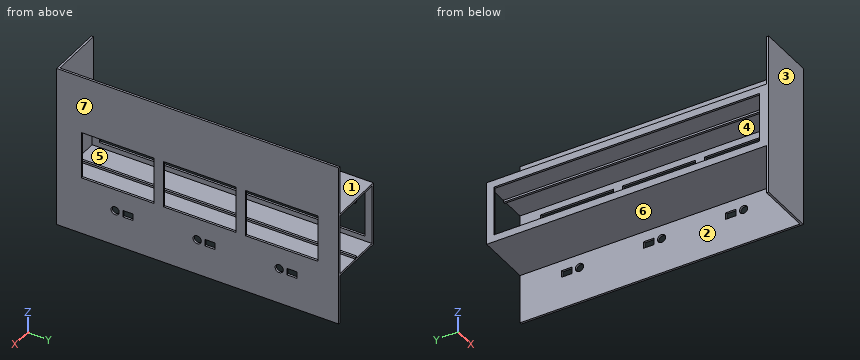
from build123d import *

# Parameters (mm, degrees)
ESQUISSE1_W             = 102
ESQUISSE1_H             = 546
BOSS_EXTRU_1_DEPTH      = 125
ESQUISSE2_W             = 117
ESQUISSE2_H             = 546
ENL_V_MAT_EXTRU_1_DEPTH = 570.3373341
ESQUISSE3_W             = 4
ESQUISSE3_H             = 546
BOSS_EXTRU_2_DEPTH      = 4
ESQUISSE4_W             = 4
ESQUISSE4_H             = 546
BOSS_EXTRU_3_DEPTH      = 4
ESQUISSE5_W             = 125
ESQUISSE5_H             = 546
BOSS_EXTRU_4_DEPTH      = 4
ESQUISSE6_W             = 97
ESQUISSE6_H             = 518
ENL_V_MAT_EXTRU_2_DEPTH = 571.067539858
ESQUISSE7_W             = 317
ESQUISSE7_H             = 546
BOSS_EXTRU_5_DEPTH      = 4
ESQUISSE8_W             = 92
ESQUISSE8_H             = 142
ENL_V_MAT_EXTRU_3_DEPTH = 600.21365138
ESQUISSE10_W            = 13.2
ESQUISSE10_H            = 20
ENL_V_MAT_EXTRU_4_DEPTH = 600.21365138
ESQUISSE12_R            = 8
ENL_V_MAT_EXTRU_5_DEPTH = 600.21365138
ESQUISSE13_W            = 110
ESQUISSE13_H            = 317
BOSS_EXTRU_6_DEPTH      = 4


with BuildPart() as part:
    # Esquisse1 → Boss.-Extru.1 (new body)
    with BuildSketch(Plane.XY):
        with Locations((51, 273)):
            Rectangle(ESQUISSE1_W, ESQUISSE1_H)
    extrude(amount=BOSS_EXTRU_1_DEPTH)

    # Esquisse2 → Enl_v. mat.-Extru.1 (cut, through all)
    with BuildSketch(Plane(origin=(102, 0, 0), x_dir=(0, 0, -1), z_dir=(1, 0, 0))):
        with Locations((-62.5, 273)):
            Rectangle(ESQUISSE2_W, ESQUISSE2_H)
    extrude(amount=-ENL_V_MAT_EXTRU_1_DEPTH, mode=Mode.SUBTRACT)


with BuildPart() as enl_v_mat_extru_1_piece_1:
    # of the separate pieces the step leaves, piece 1, a body of its own (enl_v_mat_extru_1_pieces)
    add(part.part.solids().sort_by_distance((102, 0, 121))[0])

    # Esquisse3 → Boss.-Extru.2 (add)
    with BuildSketch(Plane(origin=(0, 0, 121), x_dir=(-1, 0, 0), z_dir=(0, 0, -1))):
        with Locations((-51, 273)):
            Rectangle(ESQUISSE3_W, ESQUISSE3_H)
    extrude(amount=BOSS_EXTRU_2_DEPTH)

    # Esquisse5 → Boss.-Extru.4 (add)
    with BuildSketch(Plane.ZY):
        with Locations((62.5, 273)):
            Rectangle(ESQUISSE5_W, ESQUISSE5_H)
    extrude(amount=BOSS_EXTRU_4_DEPTH)

    # Esquisse6 → Enl_v. mat.-Extru.2 (cut, through all)
    with BuildSketch(Plane.ZY.offset(4)):
        with Locations((62.5, 273)):
            Rectangle(ESQUISSE6_W, ESQUISSE6_H)
    extrude(amount=-ENL_V_MAT_EXTRU_2_DEPTH, mode=Mode.SUBTRACT)



with BuildPart() as enl_v_mat_extru_1_piece_2:
    # of the separate pieces the step leaves, piece 2, a body of its own (enl_v_mat_extru_1_pieces)
    add(part.part.solids().sort_by_distance((0, 0, 0))[0])

    # Esquisse4 → Boss.-Extru.3 (add)
    with BuildSketch(Plane.XY.offset(4)):
        with Locations((51, 273)):
            Rectangle(ESQUISSE4_W, ESQUISSE4_H)
    extrude(amount=BOSS_EXTRU_3_DEPTH)


with BuildPart() as enl_v_mat_extru_1_piece_1_1:
    add(enl_v_mat_extru_1_piece_1.part)

    add(enl_v_mat_extru_1_piece_2.part)  # Boss.-Extru.5 merges Enl_v. mat.-Extru.1 piece 2
    # Esquisse7 → Boss.-Extru.5 (add)
    with BuildSketch(Plane(origin=(102, 0, 0), x_dir=(0, 0, -1), z_dir=(1, 0, 0))):
        with Locations((-62.5, 273)):
            Rectangle(ESQUISSE7_W, ESQUISSE7_H)
    extrude(amount=BOSS_EXTRU_5_DEPTH)

    # Esquisse8 → Enl_v. mat.-Extru.3 (cut, through all)
    with BuildSketch(Plane(origin=(106, 0, 0), x_dir=(0, 0, -1), z_dir=(1, 0, 0))):
        with Locations((-62.5, 115)):
            Rectangle(ESQUISSE8_W, ESQUISSE8_H)
        with Locations((-62.5, 275)):
            Rectangle(ESQUISSE8_W, ESQUISSE8_H)
        with Locations((-62.5, 435)):
            Rectangle(ESQUISSE8_W, ESQUISSE8_H)
    extrude(amount=-ENL_V_MAT_EXTRU_3_DEPTH, mode=Mode.SUBTRACT)

    # Esquisse10 → Enl_v. mat.-Extru.4 (cut, through all)
    with BuildSketch(Plane(origin=(106, 0, 0), x_dir=(0, 0, -1), z_dir=(1, 0, 0))):
        with Locations((26.6, 135)):
            Rectangle(ESQUISSE10_W, ESQUISSE10_H)
        with Locations((26.6, 295)):
            Rectangle(ESQUISSE10_W, ESQUISSE10_H)
        with Locations((26.6, 455)):
            Rectangle(ESQUISSE10_W, ESQUISSE10_H)
    extrude(amount=-ENL_V_MAT_EXTRU_4_DEPTH, mode=Mode.SUBTRACT)

    # Esquisse12 → Enl_v. mat.-Extru.5 (cut, through all)
    with BuildSketch(Plane(origin=(106, 0, 0), x_dir=(0, 0, -1), z_dir=(1, 0, 0))):
        with Locations((26.125, 110)):
            Circle(ESQUISSE12_R)
        with Locations((26.125, 270)):
            Circle(ESQUISSE12_R)
        with Locations((26.125, 430)):
            Circle(ESQUISSE12_R)
    extrude(amount=-ENL_V_MAT_EXTRU_5_DEPTH, mode=Mode.SUBTRACT)

    # Esquisse13 → Boss.-Extru.6 (add)
    with BuildSketch(Plane.XZ):
        with Locations((51, 62.5)):
            Rectangle(ESQUISSE13_W, ESQUISSE13_H)
    extrude(amount=BOSS_EXTRU_6_DEPTH)


solid = enl_v_mat_extru_1_piece_1_1.part
Verification items for the finished model (mm, model axes). Face numbers are marked on the shaded views. A direction names the side the tool comes from. Coordinates: 2 decimals unless noted, no trailing zeros. Order: outer loops, then holes, each group sorted by start corner. A loop starts at its lowest first (then second) coordinate and runs counter-clockwise, first axis right, second up. Notation, with made-up numbers: M -6.75,52 L 11.25,52 A22 cw 11.25,83 Z; hole C 1.25,18 d7. An arc over 180 degrees is marked long. One line per item, written item: value. Start each with the question number.
Item 1: Sectioned sample at D-D on y = 110. Give the number of separate pieces and of enclosed holes in the cut face, then the cut area to 3 significant figures.
Item 2: Access from +Z, -Z, +X, -X, +Y, -Y to the whole of each face (thin tool, end or side, straight path). Record for the marked faces 1, 2 and 3.
Item 3: Sectioned sample at A-A on y = 413. Record the cut outline in (x, z).
Item 4: Sectioned sample at C-C on x = 81. Record the cut outline in (y, z).
Item 5: Mould release check, pull along Z, two halves, no side actions. Record for the marked faces 4, 5, 6 and 7: pulls with the +Z half, pulls with the -Z half, needs draft (parallel to the pull), parting line crosses it, or undercut.
Item 6: Sectioned sample at B-B on z = 56. Record the cut outline in (x, y), then the cut area to 3 significant figures.
Item 7: Thickness scan on probe 1 along Z at (x, y) = (44, 169); probe 2 along X at (y, z) = (500, 12.5); probe 3 along X at (y, z) = (177.5, -54). Record the ranges inside material, lowest first.
Item 8: Depth check by flat-ended pin: P1, Ø24.5, axis at x = 34, y = 149, coming from the -Z side; P2, Ø4, axis at x = 75, z = 112.5, coming from the +Y side; P3, Ø3, axis at x = 94, y = 417.5, coming from the +Z side. Enter the tip coordinate at first touch or a pass-through.
Calculated:
1. separate pieces: 3
1. enclosed holes: 0
1. area: 1,800 mm^2
2. face 1: +Z, -X, +Y
2. face 2: -Z, -X, +Y
2. face 3: +Z, -Z, +X, -X, -Y
3. outline: M -4,0 L 102,0 L 102,-96 L 106,-96 L 106,16.5 L 102,16.5 L 102,4 L 53,4 L 53,8 L 49,8 L 49,4 L 0,4 L 0,14 L -4,14 Z; M -4,111 L 0,111 L 0,121 L 49,121 L 49,117 L 53,117 L 53,121 L 102,121 L 102,108.5 L 106,108.5 L 106,221 L 102,221 L 102,125 L -4,125 Z
4. outline: M -4,-96 L 0,-96 L 0,0 L 546,0 L 546,4 L 0,4 L 0,121 L 546,121 L 546,125 L 0,125 L 0,221 L -4,221 Z
5. face 4: undercut
5. face 5: undercut
5. face 6: pulls with the -Z half
5. face 7: needs draft
6. outline: M -4,-4 L 106,-4 L 106,44 L 102,44 L 102,0 L 0,0 L 0,14 L -4,14 Z; M -4,532 L 0,532 L 0,546 L -4,546 Z; M 102,186 L 106,186 L 106,204 L 102,204 Z; M 102,346 L 106,346 L 106,364 L 102,364 Z; M 102,506 L 106,506 L 106,546 L 102,546 Z
6. area: 1,030 mm^2
7. probe 1: 0 to 4, 121 to 125
7. probe 2: -4 to 0, 102 to 106
7. probe 3: 102 to 106
8. P1: z = 0
8. P2: y = 0
8. P3: z = 125
